from build123d import *

# Parameters (mm, degrees)
F2_SIZE  = 1
F4_DEPTH = 4


with BuildPart() as f1:
    # F0 (on Front) → F1 (revolve)
    with BuildSketch(Plane.XZ):
        Polygon((15, 7), (15, 0), (35, 0), (35, 4), (26, 4), (26, 7), align=None)
    revolve(axis=Axis((0, 0, 26.826651), (0, 0, 1)))

    # F2
    f2_edges = [f1.edges().sort_by_distance(p)[0] for p in [
        (-26, 0, 7),
    ]]
    chamfer(f2_edges, length=F2_SIZE)

    # F3 (on face) → F4 (cut)
    with BuildSketch(Plane.XY.offset(4)):
        with BuildLine():
            ThreePointArc((2.75, 30), (-0.063037, 32.749277), (-2.74711, 29.873958))
            ThreePointArc((-2.74711, 29.873958), (0, 27.25), (2.74711, 29.873958))
            ThreePointArc((2.74711, 29.873958), (2.749277, 29.936963), (2.75, 30))
        make_face()
        with BuildLine():
            ThreePointArc((-27.25, 0), (-28.011393, 1.899459), (-29.873958, 2.74711))
            ThreePointArc((-29.873958, 2.74711), (-32.75, 0), (-29.873958, -2.74711))
            ThreePointArc((-29.873958, -2.74711), (-28.011393, -1.899459), (-27.25, 0))
        make_face()
        with BuildLine():
            ThreePointArc((2.74711, -29.873958), (0, -27.25), (-2.74711, -29.873958))
            ThreePointArc((-2.74711, -29.873958), (-0.063037, -32.749277), (2.75, -30))
            ThreePointArc((2.75, -30), (2.749277, -29.936963), (2.74711, -29.873958))
        make_face()
        with BuildLine():
            ThreePointArc((32.75, 0), (31.899459, 1.988607), (29.873958, 2.74711))
            ThreePointArc((29.873958, 2.74711), (27.25, 0), (29.873958, -2.74711))
            ThreePointArc((29.873958, -2.74711), (31.899459, -1.988607), (32.75, 0))
        make_face()
    extrude(amount=-F4_DEPTH, mode=Mode.SUBTRACT)


solid = f1.part
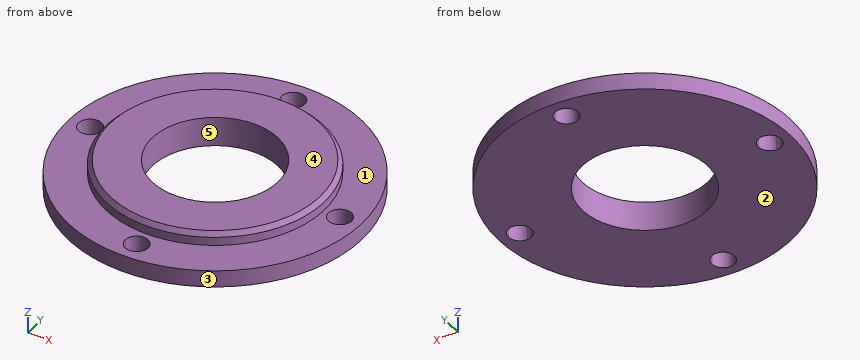
Could you check a few things on this model? Use its own coordinates, in mm. Face numbers are marked on the shaded views. A direction names the side the tool comes from. Coordinates: 2 decimals unless noted, no trailing zeros. Loops run counter-clockwise (first coordinate to the right, second up) from the corner with the lowest first, then second, coordinate; pieces in that order, holes last.
1. For the marked faces 1 and 2, which set-ups out of +Z, -Z, +X, -X, +Y, -Y let a thin tool reach every point of the face, with its end or its side?
2. Imagine slicing it at A-A (x = 0). Please give me the cut outline in (y, z).
3. I need wall thicknesses on L1, parallel to Y at x = -2, z = 1.25; L2, parallel to Z at x = -4.5, y = -29.5; L3, parallel to X at y = 28.5, z = 1. Which ranges of each line are inside material? Lowest first, please.
4. Imagine slicing it at B-B (y = 1.5). Give the number of separate pieces and of enclosed holes in the cut face, and give its area (3 significant figures).
5. For P1, Ø2, axis at x = -18, y = 27.5, coming from the +Z side; P2, Ø3, axis at y = -14.5, z = 1.5, coming from the +X side; P3, Ø1, axis at y = -12.5, z = 5, coming from the -X side, each with a flat end and sliding along its axis, tell me the tip position at first contact or that it passes through.
6. We'd pull the mould along X, two halves only. Please class the marked faces 3, 4 and 5: released by +X, released by -X, zero draft, split by the parting line, or undercut.
Computed values:
1. face 1: +Z
1. face 2: -Z, +X, -X, +Y, -Y
2. outline: (-35, 0) - (-32.75, 0) - (-32.75, 4) - (-35, 4) - close; (-27.25, 0) - (-15, 0) - (-15, 7) - (-25, 7) - (-26, 6) - (-26, 4) - (-27.25, 4) - close; (15, 0) - (27.25, 0) - (27.25, 4) - (26, 4) - (26, 6) - (25, 7) - (15, 7) - close; (32.75, 0) - (35, 0) - (35, 4) - (32.75, 4) - close
3. L1: y = -34.94 to -31.89, -28.11 to -14.87, 14.87 to 28.11, 31.89 to 34.94
3. L2: z = 0 to 4
3. L3: x = -20.32 to -2.3, 2.3 to 20.32
4. separate pieces: 4
4. enclosed holes: 0
4. area: 189 mm2
5. P1: stops at z = 4
5. P2: stops at x = 32.5
5. P3: stops at x = -23.07
6. face 3: split by the parting line
6. face 4: zero draft
6. face 5: undercut
